```python
from build123d import *

# Parameters (mm, degrees)
F1_DEPTH = 5.6642


with BuildPart() as f1:
    # F0 (on Top) → F1 (new body)
    with BuildSketch(Plane.XY):
        with BuildLine():
            Line((-44.324736, 2.5019), (-44.324736, 3.135164))
            ThreePointArc((-44.324736, 3.135164), (-47.4599, 0), (-44.324736, -3.135164))
            Line((-44.324736, -3.135164), (-44.324736, -2.5019))
            ThreePointArc((-44.324736, -2.5019), (-46.826636, 0), (-44.324736, 2.5019))
        make_face()
        with BuildLine():
            ThreePointArc((-41.189572, 0), (-42.10784, 2.216896), (-44.324736, 3.135164))
            Line((-44.324736, 3.135164), (-44.324736, 2.5019))
            ThreePointArc((-44.324736, 2.5019), (-42.555625, 1.76911), (-41.822836, 0))
            ThreePointArc((-41.822836, 0), (-42.555625, -1.76911), (-44.324736, -2.5019))
            Line((-44.324736, -2.5019), (-44.324736, -3.135164))
            ThreePointArc((-44.324736, -3.135164), (-42.10784, -2.216896), (-41.189572, 0))
        make_face()
        with BuildLine():
            Line((44.324736, 3.135164), (-44.324736, 3.135164))
            ThreePointArc((-44.324736, 3.135164), (-42.10784, 2.216896), (-41.189572, 0))
            ThreePointArc((-41.189572, 0), (-42.10784, -2.216896), (-44.324736, -3.135164))
            Line((-44.324736, -3.135164), (44.324736, -3.135164))
            ThreePointArc((44.324736, -3.135164), (41.189572, 0), (44.324736, 3.135164))
        make_face()
        with BuildLine():
            ThreePointArc((47.4599, 0), (46.541632, 2.216896), (44.324736, 3.135164))
            Line((44.324736, 3.135164), (44.324736, 2.5019))
            ThreePointArc((44.324736, 2.5019), (46.093846, 1.76911), (46.826636, 0))
            ThreePointArc((46.826636, 0), (46.093846, -1.76911), (44.324736, -2.5019))
            Line((44.324736, -2.5019), (44.324736, -3.135164))
            ThreePointArc((44.324736, -3.135164), (46.541632, -2.216896), (47.4599, 0))
        make_face()
        with BuildLine():
            Line((44.324736, 2.5019), (44.324736, 3.135164))
            ThreePointArc((44.324736, 3.135164), (41.189572, 0), (44.324736, -3.135164))
            Line((44.324736, -3.135164), (44.324736, -2.5019))
            ThreePointArc((44.324736, -2.5019), (41.822836, 0), (44.324736, 2.5019))
        make_face()
    extrude(amount=F1_DEPTH)


solid = f1.part
```
Source: CAD feature listing. Evaluate the final solid. Frame: model axes, mm. Round coordinates to 2 decimals unless told otherwise and drop trailing zeros. Loops run counter-clockwise (first coordinate to the right, second up) from the corner with the lowest first, then second, coordinate; pieces in that order, holes last.
(1) Section query A-A (z = 2.35). Output: boundary loops of the cut face in (x, y), and give its area (3 significant figures).
From the geometry:
outline: (-44.32, -3.14) - (44.32, -3.14) arc R3.14 ccw to (47.46, 0) arc R3.14 ccw to (44.32, 3.14) - (-44.32, 3.14) arc R3.14 ccw to start; hole circle Ø5 at (-44.32, 0); hole (44.32, -2.5) arc R2.5 ccw to (46.83, 0) arc R2.5 ccw to (44.32, 2.5) arc R2.5 ccw to start
area: 547 mm2
(2) Section query B-B (y = 1.5). Output: boundary loops of the cut face in (x, z), and give its area (3 significant figures).
From the geometry:
outline: (-47.08, 0) - (-46.33, 0) - (-46.33, 5.66) - (-47.08, 5.66) - close; (-42.32, 0) - (42.32, 0) - (42.32, 5.66) - (-42.32, 5.66) - close; (46.33, 0) - (47.08, 0) - (47.08, 5.66) - (46.33, 5.66) - close
area: 488 mm2
(3) Material intervals for probe 1 along X at (y, z) = (1, 1.35); probe 2 along X at (y, z) = (1.5, 3.9), sorted ascending.
From the geometry:
probe 1: x = -47.3 to -46.62, -42.03 to 42.03, 46.62 to 47.3
probe 2: x = -47.08 to -46.33, -42.32 to 42.32, 46.33 to 47.08
(4) Contact query for a flat-ended pin moving along its axis: pin 1 Ø2 at (y, z) = (2, 2.5) entering from +X. Output: stop coordinate, or through.
From the geometry:
pin 1: stops at x = 47.3
